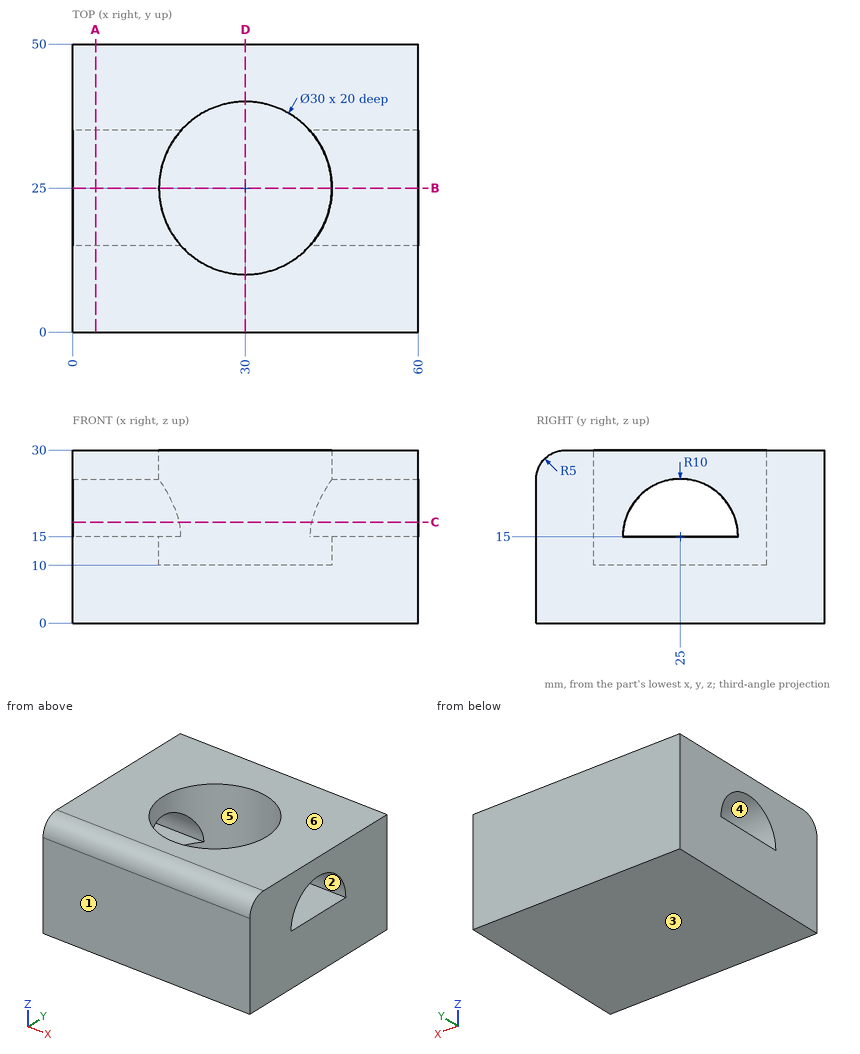
Study the drawing (mm; zero at the part's minimum x, y, z) and answer. A direction names the side the tool comes from. Coordinates: 2 decimals unless noted, no trailing zeros. Loops run counter-clockwise (first coordinate to the right, second up) from the corner with the lowest first, then second, coordinate; pieces in that order, holes last. Notation, with made-up numbers: (15.25, 44) -> (60.25, 44) arc R18 ccw to (60.25, 54) -> close; hole circle Ø1 at (12.25, 9). An arc over 180 degrees is marked (long way). Answer in a Markdown table with one row per item. Add a question column.
1. The part is cut by section D-D, the plane x = 30. Write down the section's boundary in (y, z), then the cut area to 3 significant figures.
2. The part is cut by section A-A, the plane x = 4. Write down the section's boundary in (y, z).
3. A flat-ended cylindrical pin translates along its axis: P1, Ø9, axis at x = 27, y = 24, coming from the +Z side. Find the tip coordinate at first contact, or state that the pin passes through.
4. Consider line 1 (Y direction, x = 30, z = 19.5); line 2 (X direction, y = 32.5, z = 22); line 3 (Z direction, x = 38, y = 22.5). Determine where each line is inside the solid, lowest interval first. Write a range as [from, to].
5. For the marked faces 4, 5 and 6, determine the directions among +Z, -Z, +X, -X, +Y, -Y from which every point of the face is accessible in a straight line to the end or side of a thin tool.
6. The part is cut by section B-B, the plane y = 25. Write down the section's boundary in (x, z), then the cut area to 3 significant figures.
7. Determine the mould class of the marked faces 1, 2 and 3 for opening direction Z: +Z half, -Z half, draft (parallel to the pull), parting line (faces both ways), or undercut.
8. The part is cut by section C-C, the plane z = 17.5. Write down the section's boundary in (x, y).
Answer below:
| question | item | result |
|---|---|---|
| 1 | outline | (0, 0) -> (50, 0) -> (50, 30) -> (40, 30) -> (40, 10) -> (10, 10) -> (10, 30) -> (5, 30) arc R5 ccw to (0, 25) -> close |
| 1 | area | 895 mm2 |
| 2 | outline | (0, 0) -> (50, 0) -> (50, 30) -> (5, 30) arc R5 ccw to (0, 25) -> close; hole (15, 15) -> (35, 15) arc R10 ccw to start |
| 3 | P1 | z = 10 |
| 4 | line 1 | [0, 10], [40, 50] |
| 4 | line 2 | [0, 17.01], [42.99, 60] |
| 4 | line 3 | [0, 10] |
| 5 | face 4 | +X, -X |
| 5 | face 5 | +Z |
| 5 | face 6 | +Z, +X, -X, +Y, -Y |
| 6 | outline | (0, 0) -> (60, 0) -> (60, 15) -> (45, 15) -> (45, 10) -> (15, 10) -> (15, 15) -> (0, 15) -> close; (0, 25) -> (15, 25) -> (15, 30) -> (0, 30) -> close; (45, 25) -> (60, 25) -> (60, 30) -> (45, 30) -> close |
| 6 | area | 900 mm2 |
| 7 | face 1 | draft |
| 7 | face 2 | undercut |
| 7 | face 3 | -Z half |
| 8 | outline | (0, 0) -> (60, 0) -> (60, 15.32) -> (41.46, 15.32) arc R15 cw to (18.54, 15.32) -> (0, 15.32) -> close; (0, 34.68) -> (18.54, 34.68) arc R15 cw to (41.46, 34.68) -> (60, 34.68) -> (60, 50) -> (0, 50) -> close |
